from build123d import *

# Parameters (mm, degrees)
F2_DEPTH   = 25.4
F3_SIZE2   = 4.022955
F3_SIZE    = 25.39999
F3_2_SIZE2 = 4.022955
F3_2_SIZE  = 25.39999


# Not quite as in the source:
# - a fillet or chamfer is up to 0.001 mm smaller than in the source, because OpenCascade refuses the exact size


with BuildPart() as f2:
    # F1 (on Top) → F2 (new body)
    with BuildSketch(Plane.XY):
        Polygon((-122.5808599955, 457.2), (-25.4, 0), (25.4, 0), (122.5808599955, 457.2), align=None)
    extrude(amount=F2_DEPTH)

    # F3 (size 25.4 and 4.0229647842 in the source; OpenCascade refuses exactly that, so slightly less here)
    f3_edges = [f2.edges().sort_by_distance(p)[0] for p in [
        (-73.99043, 228.6, 25.4),
    ]]
    f3_side = f2.faces().sort_by_distance((-73.99043, 228.6, 12.7))[0]
    chamfer(f3_edges, length=F3_SIZE, length2=F3_SIZE2, reference=f3_side)

    # F3#2 (size 25.4 and 4.0229647842 in the source; OpenCascade refuses exactly that, so slightly less here)
    f3_2_edges = [f2.edges().sort_by_distance(p)[0] for p in [
        (73.99043, 228.6, 25.4),
    ]]
    f3_2_side = f2.faces().sort_by_distance((73.99043, 228.6, 12.7))[0]
    chamfer(f3_2_edges, length=F3_2_SIZE, length2=F3_2_SIZE2, reference=f3_2_side)


solid = f2.part
Geometry check sheet. Reference: the model listing, model coordinates, mm. Give positions to 0.01 mm unless a question says otherwise; leave off trailing zeros. Loops run counter-clockwise (first coordinate to the right, second up) from the corner with the lowest first, then second, coordinate; pieces in that order, holes last. Notation, with made-up numbers: (15.25, -33.5) -> (53.25, -33.5) arc R7 cw to (53.25, -28.5) -> close; hole circle Ø4 at (45.5, 2). An arc over 180 degrees is marked (long way). Answer in a Markdown table with one row per item. Add a question column.
1) Material ranges on probe 1 along X at (y, z) = (255, 21.25); probe 2 along X at (y, z) = (73, 18.75), recorded low to high. Write a range as from..to.
2) Gauge pin test, flat ends, axial feed: P1, Ø3, axis at y = 130.5, z = 21, coming from the -X side; P2, Ø8, axis at y = 130, z = 8.5, coming from the -X side; P3, Ø6, axis at y = 54, z = 17, coming from the +X side. Record the tip position at first contact, or that the pin passes through.
3) Cross-section at C-C on z = 15. Record the boundary of the cut face in (x, y), and give its area (3 significant figures).
Outcome:
| question | item | result |
|---|---|---|
| 1 | probe 1 | x = -76.16..76.16 |
| 1 | probe 2 | x = -37.88..37.88 |
| 2 | P1 | stops at x = -50.14 |
| 2 | P2 | stops at x = -52.72 |
| 2 | P3 | stops at x = 34.93 |
| 3 | outline | (-120.15, 457.2) -> (-22.97, 0) -> (22.97, 0) -> (120.15, 457.2) -> close |
| 3 | area | 65,400 mm^2 |
